```python
from build123d import *

# Parameters (mm, degrees)
SKETCH1_R           = 1.7
BOSS_EXTRUDE1_DEPTH = 12
SKETCH2_R           = 1.7
BOSS_EXTRUDE2_DEPTH = 6.2125


with BuildPart() as part:
    # Sketch1 → Boss-Extrude1 (new body)
    with BuildSketch(Plane(origin=(0, 0, 0), x_dir=(1, 0, 0), z_dir=(0, 1, 0))):
        Polygon((-10.15, 81.202952909), (10.15, 81.202952909), (10.15, -53.848636554), (16.06, -53.848636554), (16.06, -65.254427144), (6.15, -65.254427144), (6.15, -66.934427144), (-6.15, -66.934427144), (-6.15, -65.254427144), (-16.06, -65.254427144), (-16.06, -54.004427144), (-10.15, -54.004427144), align=None)
        with Locations(Location((5.4, 57.504034689, 0), (0, 0, 270))):
            Circle(SKETCH1_R, mode=Mode.SUBTRACT)
        with Locations(Location((5.4, 30.504034689, 0), (0, 0, 270))):
            Circle(SKETCH1_R, mode=Mode.SUBTRACT)
        with Locations(Location((5.4001, 53.054034689, 0), (0, 0, 270))):
            Circle(SKETCH1_R, mode=Mode.SUBTRACT)
        with Locations(Location((5.4001, 26.054034689, 0), (0, 0, 270))):
            Circle(SKETCH1_R, mode=Mode.SUBTRACT)
        with Locations(Location((5.4, 61.954034689, 0), (0, 0, 270))):
            Circle(SKETCH1_R, mode=Mode.SUBTRACT)
        with Locations(Location((5.39995, 34.954034689, 0), (0, 0, 270))):
            Circle(SKETCH1_R, mode=Mode.SUBTRACT)
        with Locations(Location((5.4, 48.60403469, 0), (0, 0, 270))):
            Circle(SKETCH1_R, mode=Mode.SUBTRACT)
        with Locations(Location((5.40005, 66.404034689, 0), (0, 0, 270))):
            Circle(SKETCH1_R, mode=Mode.SUBTRACT)
        with Locations(Location((5.4, 21.60403469, 0), (0, 0, 270))):
            Circle(SKETCH1_R, mode=Mode.SUBTRACT)
        with Locations(Location((5.4, 39.404034689, 0), (0, 0, 270))):
            Circle(SKETCH1_R, mode=Mode.SUBTRACT)
    extrude(amount=BOSS_EXTRUDE1_DEPTH)

    # Sketch2 → Boss-Extrude2 (add, symmetric)
    with BuildSketch(Plane(origin=(0, 0, 0), x_dir=(0, 0, -1), z_dir=(1, 0, 0))):
        with BuildLine():
            Line((-72.207292933, 5.999665069), (-72.207292933, 8.809665069))
            ThreePointArc((-72.207292933, 8.809665069), (-70.110812417, 11.254776949), (-66.977292933, 11.999665069))
            Line((-66.977292933, 11.999665069), (-66.934427144, 12))
            Line((-66.934427144, 12), (-66.934427144, 0))
            Line((-66.934427144, 0), (-72.207292933, 0))
            Line((-72.207292933, 0), (-72.207292933, 5.999665069))
        make_face()
        with Locations((-69.217292933, 8.579665069)):
            Circle(SKETCH2_R, mode=Mode.SUBTRACT)
    extrude(amount=BOSS_EXTRUDE2_DEPTH, both=True)


solid = part.part
```
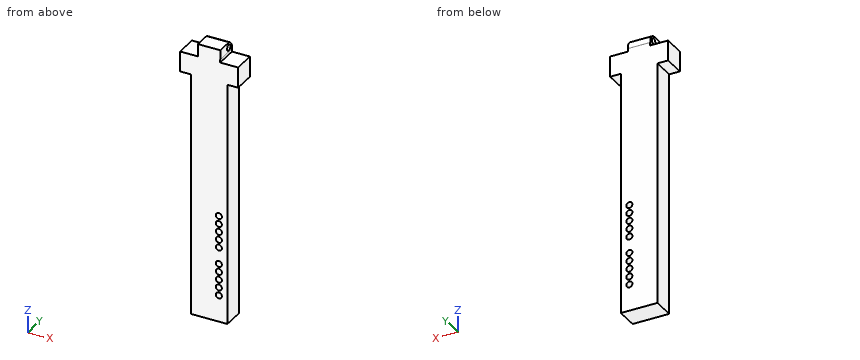
Check sheet for the modelled part. Datum: model origin and axes. Units: mm. Round coordinates to 2 decimals unless told otherwise and drop trailing zeros. Loops run counter-clockwise (first coordinate to the right, second up) from the corner with the lowest first, then second, coordinate; pieces in that order, holes last. Notation, with made-up numbers: (32.5, 35.25) - (87.5, 35.25) arc R16 cw to (87.5, 39.25) - close; hole circle Ø7 at (-34.5, 84). An arc over 180 degrees is marked (long way). Write item = value, one per line. Start each with the question number.
Q1. Section check B-B (y = 2.75). Count the separate pieces of the cut face and the enclosed holes in it, plus the area to 3 significant figures.
Q2. Thickness scan on L1, parallel to X at y = 6, z = -57.5; L2, parallel to Y at x = -5, z = 39.5; L3, parallel to X at y = 6.5, z = 39. Record the ranges inside material, lowest first.
Q3. Section check C-C (x = 13.5). Record the boundary of the cut face in (y, z).
Q4. Depth check by flat-ended pin: P1, Ø5, axis at x = 12.5, y = 3.5, coming from the +Z side; P2, Ø6, axis at y = 4, z = 69, coming from the -X side; P3, Ø1.5, axis at x = 12.5, z = -29, coming from the +Y side; P4, Ø3.5, axis at y = 7.5, z = 3, coming from the -X side. Enter the tip coordinate at first touch or a pass-through.
Q5. Section check A-A (z = 49.5). Record the boundary of the cut face in (x, y), plus the area to 3 significant figures.
Derived:
q1.separate_pieces = 1
q1.enclosed_holes = 10
q1.area = 3,100 mm^2
q2.L1 = -10.15 to 3.7, 7.1 to 10.15
q2.L2 = 0 to 12
q2.L3 = -10.15 to 10.15
q3.outline = (0, 53.85) - (12, 53.85) - (12, 65.25) - (0, 65.25) - close
q4.P1 = 65.25
q4.P2 = -6.21
q4.P3 = through
q4.P4 = -10.15
q5.outline = (-10.15, 0) - (10.15, 0) - (10.15, 12) - (-10.15, 12) - close
q5.area = 244 mm^2
